Part model, mm, in its own coordinate system. Face numbers are marked on the shaded views. Round coordinates to 2 decimals unless told otherwise and drop trailing zeros. Write each loop counter-clockwise with the first axis right and the second up, starting at its lowest first coordinate (ties: lowest second). Pieces come first, ordered by that corner, then holes. Notation, with made-up numbers: M 30.5,-35 L 82.5,-35 A14 cw 82.5,-25 Z; hole C 54.5,-4 d11. An arc over 180 degrees is marked long. One line per question, with ' | ' between items. Start each with the question number.
1) Saw through at B-B (z = 0). Give the number of separate pieces and of enclosed holes in the cut face, plus the area to 3 significant figures.
2) Saw through at C-C (y = -8). List the corners of the cut face in (x, z), plus the area to 3 significant figures.
3) Mould opens along Y. For the marked faces 1, 2 and 3 say: pulls with the +Y half, pulls with the -Y half, needs draft (parallel to the pull), parting line crosses it, or undercut.
4) Saw through at D-D (x = 12.5). List the corners of the cut face in (y, z), plus the area to 3 significant figures.
5) Wall check: probe 1 along X at (y, z) = (-37, -44.5); probe 2 along Z at (x, y) = (-0.5, -10.5); probe 3 along Y at (x, z) = (8, 3.5). Give the ranges that are in metal, low to high. Write a range as [from, to].
6) Saw through at A-A (x = 21.75). List the corners of the cut face in (y, z), plus the area to 3 significant figures.
7) Drop flat-ended pins along their axis: pin 1 Ø12 at (x, y) = (8, 55) entering from +Z; pin 2 Ø3.5 at (y, z) = (44.19, 44.19) entering from -X; pin 3 Ø3 at (y, z) = (-46.5, 43.5) entering from +X; pin 4 Ø3.5 at (x, y) = (20, 11.5) entering from +Z. Give the stop position or say it passes through.
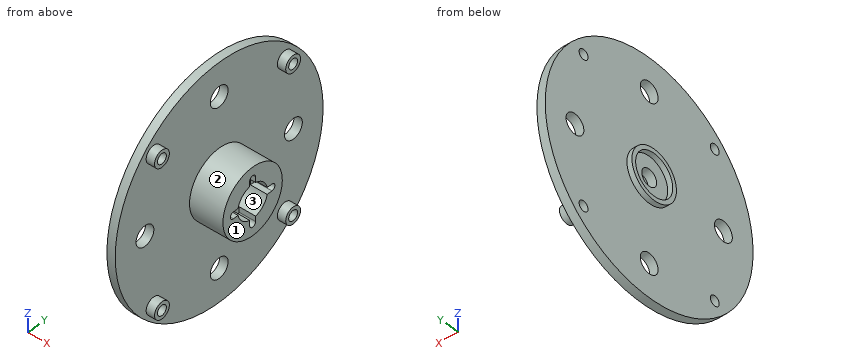
Autodesk Inventor part; units mm, degrees
ref_plane "Lock Pin Hole Plane" through (0, 15.875, 0) normal (0, 1, 0) x (-1, 0, 0)
ref_plane "YZ Plane" through (0, 0, 0) normal (1, 0, 0) x (0, 1, 0)
ref_plane "XY Plane" through (0, 0, 0) normal (0, 0, 1) x (1, 0, 0)
sketch "Sketch1" plane through (0, 0, 0) normal (1, 0, 0) x (0, 1, 0)
  circle A0 centre (0, 0) radius 70
  dimension "d2" = 140
extrude "Hub Face" add sketch "Sketch1" along normal blind 5
sketch "Sketch2" plane through (5, 0, 0) normal (1, 0, 0) x (0, 0, -1)
  circle A0 centre (0, 0) radius 50 construction
  circle A1 centre (0, 50) radius 6
  line L0 (0, 50) -> (0, 0) construction
  dimension "d4" = 100
  dimension "d3" = 12
extrude "Lug Bolt Hole" cut sketch "Sketch2" against normal up to surface (5 mm away)
pattern_circular "Lug Bolt Hole Pattern" count 4 over 360 about axis through (-10, 0, 0) along (1, 0, 0) of "Lug Bolt Hole"
sketch "Sketch3" plane through (5, 0, 0) normal (1, 0, 0) x (0, 0, -1)
  circle A0 centre (0, 0) radius 20
  circle A1 centre (0, 0) radius 10
  line L0 (-98, 0) -> (98, 0) construction
  line L1 (0, -98) -> (0, 98) construction
  arc A2 (13, -2) -> (13, 2) centre (13, 0) ccw
  arc A3 (7, 2) -> (7, -2) centre (7, 0) ccw
  line L2 (13, 2) -> (7, 2)
  line L3 (13, -2) -> (7, -2)
  point P0 (10, 0)
  point P1 (9.798, -2)
  point P2 (9.798, 2)
  dimension "d19" = 20
  dimension "d10" = 40
  dimension "d59" = 6
  dimension "d60" = 2
  dimension "d61" = 7
  dimension "d62" = 3
  dimension "d63" = 3
extrude "Hub Shaft" add sketch "Sketch3" along normal blind 20 contours A0 | A1 L2 A2 L3
ref_plane "Lock Pin Hole Plane" through (0, 15.875, 0) normal (0, 1, 0) x (-1, 0, 0)
sketch "Sketch10" plane through (25, 0, 0) normal (1, 0, 0) x (0, 0, -1)
  line L0 (-98, 0) -> (98, 0) construction
  arc A0 (7, 2) -> (7, -2) centre (7, 0) ccw
  line L1 (13, 2) -> (7, 2)
  line L2 (13, -2) -> (7, -2)
  arc A1 (13, -2) -> (13, 2) centre (13, 0) ccw
  point P0 (0, 0)
  dimension "d75" = 6
  dimension "d76" = 2
extrude "Key Slot" cut sketch "Sketch10" against normal blind 10
pattern_circular "Key Slot Pattern" count 4 over 360 about axis through (-10, 0, 0) along (1, 0, 0) of "Key Slot"
sketch "Sketch12" plane through (5, 0, 0) normal (1, 0, 0) x (0, 0, -1)
  arc A0 (-2, 9.798) -> (-9.798, 2) centre (0, 0) ccw construction
  arc A1 (-9.798, -2) -> (-2, -9.798) centre (0, 0) ccw construction
  arc A2 (2, -9.798) -> (9.798, -2) centre (0, 0) ccw construction
  arc A3 (9.798, 2) -> (2, 9.798) centre (0, 0) ccw construction
  circle A4 centre (0, 0) radius 10 construction
  circle A5 centre (0, 0) radius 10
  circle A6 centre (0, 0) radius 5
  dimension "d74" = 10
extrude "Extrusion10" cut sketch "Sketch12" against normal through all contours A6
sketch "Sketch13" plane through (0, 0, 0) normal (-1, 0, 0) x (0, 0, 1)
  circle A0 centre (0, 0) radius 15
  circle A1 centre (0, 0) radius 12.5
  dimension "d77" = 30
  dimension "d78" = 25
extrude "Extrusion11" add sketch "Sketch13" along normal blind 3
sketch "Sketch14" plane through (5, 0, 0) normal (1, 0, 0) x (0, 0, -1)
  circle A0 centre (0, 0) radius 62.5 construction
  circle A1 centre (44.1942, 44.1942) radius 5
  line L0 (-98, 0) -> (98, 0) construction
  line L1 (0, -98) -> (0, 98) construction
  line L2 (0, 0) -> (44.1942, 44.1942) construction
  circle A2 centre (44.1942, 44.1942) radius 3
  dimension "d81" = 125
  dimension "d82" = 45
  dimension "d83" = 10
  dimension "d84" = 6
extrude "Extrusion12" add sketch "Sketch14" along normal blind 5
extrude "Extrusion13" cut sketch "Sketch14" against normal through all contours A2
pattern_circular "Circular Pattern6" count 4 over 360 about axis through (-10, 0, 0) along (1, 0, 0) of "Extrusion12", "Extrusion13"
equation "\"d2\" = Hub_Diameter"
equation "\"d0\" = Hub_Thickness"
equation "\"d4\" = Lug_Bolt_Pattern_Diameter"
equation "\"d3\" = Lug_Bolt_Hole_Diameter"
equation "\"d17\" = Hub_Shaft_Length"
equation "\"Hub_Thickness\" = 5"
equation "\"Hub_Diameter\" = 140"
equation "\"Lug_Bolt_Hole_Diameter\" = 12"
equation "\"Hub_Shaft_Diameter\" = 1"
equation "\"Hub_Shaft_Wall_Thickness\" = 1"
equation "\"Hub_Shaft_Length\" = 20"
equation "\"Hub_Shaft_Outer_Diameter\" = 31.75"
equation "\"d20\" = 0.5 * Hub_Shaft_Outer_Diameter"
equation "\"Lock_Pin_Edge_Distance\" = 15"
equation "\"Wheel_Center_Hub_Diameter_Wall_Thickness\" = 5"
equation "\"Wheel_Center_Hub_Length\" = 5"
equation "\"Weight_Reduction_Hole_Angle\" = 45deg"
properties part number "Hub"
Answer key:
1) separate pieces: 4 | enclosed holes: 0 | area: 845 mm2
2) outline: M -3,-12.69 L 0,-12.69 L 0,-69.54 L 5,-69.54 L 5,-18.33 L 25,-18.33 L 25,-6 L 5,-6 L 5,6 L 25,6 L 25,18.33 L 5,18.33 L 5,69.54 L 0,69.54 L 0,12.69 L -3,12.69 L -3,9.6 L 0,9.6 L 0,-9.6 L -3,-9.6 Z | area: 1,210 mm2
3) face 1: needs draft | face 2: parting line crosses it | face 3: undercut
4) outline: C 0,0 d40; hole C 0,0 d20 | area: 942 mm2
5) probe 1: x = [0, 5] | probe 2: z = [-10.71, -6.78], [6.78, 10.71] | probe 3: y = [-19.69, -9.37], [9.37, 19.69]
6) outline: C 0,0 d40; hole M -13,-2 L -9.8,-2 A10 ccw -2,-9.8 L -2,-13 A2 ccw 2,-13 L 2,-9.8 A10 ccw 9.8,-2 L 13,-2 A2 ccw 13,2 L 9.8,2 A10 ccw 2,9.8 L 2,13 A2 ccw -2,13 L -2,9.8 A10 ccw -9.8,2 L -13,2 A2 ccw Z | area: 868 mm2
7) pin 1: stops at z = 49.19 | pin 2: passes through | pin 3: stops at x = 10 | pin 4: stops at z = 17.46
